from build123d import *

# Parameters (mm, degrees)
SKETCH1_R           = 1.984375
SKETCH1_R_2         = 3.175
SKETCH1_R_3         = 10.0000054
SKETCH1_R_4         = 86.7075
BOSS_EXTRUDE1_DEPTH = 3.175


with BuildPart() as part:
    # Sketch1 → Boss-Extrude1 (new body)
    with BuildSketch(Plane.XZ.offset(64.8)):
        with BuildLine():
            ThreePointArc((-35.802288852, -190.105967461), (0, -215.175), (35.802288852, -190.105967461))
            Line((35.802288852, -190.105967461), (45.31324895, -163.974819355))
            ThreePointArc((45.31324895, -163.974819355), (66.095055559, -119.40809126), (94.300070948, -79.127154752))
            ThreePointArc((94.300070948, -79.127154752), (0, 123.1), (-94.300070948, -79.127154752))
            ThreePointArc((-94.300070948, -79.127154752), (-66.095055559, -119.40809126), (-45.31324895, -163.974819355))
            Line((-45.31324895, -163.974819355), (-35.802288852, -190.105967461))
        make_face()
        with Locations(Location((-17.960512242, -195.035512242, 0), (0, 0, 270))):
            Circle(SKETCH1_R, mode=Mode.SUBTRACT)
        with Locations(Location((-47.329330924, -142.15, 0), (0, 0, 270))):
            Circle(SKETCH1_R_2, mode=Mode.SUBTRACT)
        with Locations(Location((-17.960512242, -159.114487758, 0), (0, 0, 270))):
            Circle(SKETCH1_R, mode=Mode.SUBTRACT)
        with Locations(Location((-82.554716704, -82.554716704, 0), (0, 0, 270))):
            Circle(SKETCH1_R_2, mode=Mode.SUBTRACT)
        with Locations(Location((-25.4, -119.925, 0), (0, 0, 270))):
            Circle(SKETCH1_R_2, mode=Mode.SUBTRACT)
        with Locations(Location((0, -208.825, 0), (0, 0, 270))):
            Circle(SKETCH1_R_2, mode=Mode.SUBTRACT)
        with Locations(Location((17.960512242, -195.035512242, 0), (0, 0, 270))):
            Circle(SKETCH1_R, mode=Mode.SUBTRACT)
        with Locations(Location((0, -177.075, 0), (0, 0, 270))):
            Circle(SKETCH1_R_3, mode=Mode.SUBTRACT)
        with Locations(Location((17.960512242, -159.114487758, 0), (0, 0, 270))):
            Circle(SKETCH1_R, mode=Mode.SUBTRACT)
        with Locations(Location((47.329330924, -142.15, 0), (0, 0, 270))):
            Circle(SKETCH1_R_2, mode=Mode.SUBTRACT)
        with Locations(Location((25.4, -119.925, 0), (0, 0, 270))):
            Circle(SKETCH1_R_2, mode=Mode.SUBTRACT)
        with Locations(Location((82.554716704, -82.554716704, 0), (0, 0, 270))):
            Circle(SKETCH1_R_2, mode=Mode.SUBTRACT)
        with Locations(Location((-116.75, 0, 0), (0, 0, 270))):
            Circle(SKETCH1_R_2, mode=Mode.SUBTRACT)
        with Locations(Location((-82.554716704, 82.554716704, 0), (0, 0, 270))):
            Circle(SKETCH1_R_2, mode=Mode.SUBTRACT)
        with Locations(Location((0, 116.75, 0), (0, 0, 270))):
            Circle(SKETCH1_R_2, mode=Mode.SUBTRACT)
        with Locations(Location((116.75, 0, 0), (0, 0, 270))):
            Circle(SKETCH1_R_2, mode=Mode.SUBTRACT)
        with Locations(Location((82.554716704, 82.554716704, 0), (0, 0, 270))):
            Circle(SKETCH1_R_2, mode=Mode.SUBTRACT)
        with Locations(Location((66.026095693, 66.026095693, 0), (0, 0, 270))):
            Circle(SKETCH1_R_2, mode=Mode.SUBTRACT)
        with Locations(Location((-66.026095693, -66.026095693, 0), (0, 0, 270))):
            Circle(SKETCH1_R_2, mode=Mode.SUBTRACT)
        with Locations(Location((66.026095693, -66.026095693, 0), (0, 0, 270))):
            Circle(SKETCH1_R_2, mode=Mode.SUBTRACT)
        with Locations(Location((-66.026095693, 66.026095693, 0), (0, 0, 270))):
            Circle(SKETCH1_R_2, mode=Mode.SUBTRACT)
        with Locations(Location((0, 0, 0), (0, 0, 270))):
            Circle(SKETCH1_R_4, mode=Mode.SUBTRACT)
    extrude(amount=BOSS_EXTRUDE1_DEPTH)


solid = part.part
Could you check a few things on this model? Use its own coordinates, in mm. Give positions to 0.01 mm unless a question says otherwise; leave off trailing zeros. Write each loop counter-clockwise with the first axis right and the second up, starting at its lowest first coordinate (ties: lowest second). Pieces come first, ordered by that corner, then holes. Notation, with made-up numbers: (-0.5, 4) -> (20.5, 4) arc R33 ccw to (20.5, 41) -> close; hole circle Ø4 at (61, 64.25). An arc over 180 degrees is marked (long way). Answer as a JSON object with one key per item and string values.
Q1. We'd pull the mould along X, two halves only. Please class faces 1 (the cylindrical face through (-24.446, -66.365, -122.953)), 2 (the cylindrical face through (-65.9, -66.4, 69.2)), 3 (the cylindrical face through (-66.44, -66.37, -118.81)), 4 (the flat face through (-56, -64.8, -81)): released by +X, released by -X, zero draft, split by the parting line, or undercut.
Taken from the geometry:
{"face 1": "undercut", "face 2": "undercut", "face 3": "released by -X", "face 4": "zero draft"}
Q2. Suppose I cut it at C-C on y = -65.85. Count the separate pieces of the cut face and the enclosed holes in it, then the cut area to 3 significant figures.
Taken from the geometry:
{"separate pieces": "1", "enclosed holes": "22", "area": "32,100 mm²"}
Q3. Will these pins go through, and if not, where does the flat tip stop? pin 1 Ø4 at (x, z) = (82.55, 82.55) entering from -Y; pin 2 Ø1.5 at (y, z) = (-67, 62.5) entering from +X; pin 3 Ø1 at (x, y) = (-89, -65) entering from -Z; pin 4 Ø1.5 at (y, z) = (-67.5, -88.5) entering from +X.
Taken from the geometry:
{"pin 1": "passes through", "pin 2": "stops at x = 106.49", "pin 3": "stops at z = -86.27", "pin 4": "stops at x = 87.35"}
Q4. Please list where these lines run through material, in increasing order: L1, parallel to X at y = -66.3, z = 0 (1 decimal); L2, parallel to X at y = -66.45, z = -142.15; L3, parallel to Z at x = 6, y = -67.5 (3 decimals).
Taken from the geometry:
{"L1": "x = -123.1 to -119.9, -113.6 to -86.7, 86.7 to 113.6, 119.9 to 123.1", "L2": "x = -54.31 to -50.5, -44.15 to 44.15, 50.5 to 54.31", "L3": "z = -214.7 to -185.075, -169.075 to -86.5, 86.5 to 122.954"}
Q5. Suppose I cut it at B-B on z = -40. Write out the boundary of the cut face in (x, y) (3 decimals), then the cut area to 3 significant figures.
Taken from the geometry:
{"outline": "(-116.42, -67.975) -> (-76.93, -67.975) -> (-76.93, -64.8) -> (-116.42, -64.8) -> close; (76.93, -67.975) -> (116.42, -67.975) -> (116.42, -64.8) -> (76.93, -64.8) -> close", "area": "251 mm²"}
Q6. Suppose I cut it at D-D on z = -131.5. Write out the boundary of the cut face in (x, y) (3 decimals).
Taken from the geometry:
{"outline": "(-59.502, -67.975) -> (59.502, -67.975) -> (59.502, -64.8) -> (-59.502, -64.8) -> close"}
Q7. Suppose I cut it at A-A on x = 39.5. Write out the boundary of the cut face in (y, z) (3 decimals).
Taken from the geometry:
{"outline": "(-67.975, -179.947) -> (-64.8, -179.947) -> (-64.8, -77.188) -> (-67.975, -77.188) -> close; (-67.975, 77.188) -> (-64.8, 77.188) -> (-64.8, 116.591) -> (-67.975, 116.591) -> close"}
